```python
from build123d import *

# Parameters (mm, degrees)
SKETCH1_R           = 18
BOSS_EXTRUDE1_DEPTH = 1.5
SKETCH2_R           = 17.5
BOSS_EXTRUDE2_DEPTH = 1.5
SKETCH3_R           = 12
BOSS_EXTRUDE3_DEPTH = 1
SKETCH4_R           = 10.5
BOSS_EXTRUDE4_DEPTH = 12
SKETCH5_R           = 9.5
BOSS_EXTRUDE5_DEPTH = 1
SKETCH6_R           = 10.5
BOSS_EXTRUDE6_DEPTH = 1
SKETCH8_R           = 2.705
CUT_EXTRUDE1_DEPTH  = 32.176914536
SKETCH9_R           = 7
SKETCH9_R_2         = 5
CUT_EXTRUDE3_DEPTH  = 4
SKETCH10_R          = 1.4
CUT_EXTRUDE4_DEPTH  = 5
CIRPATTERN1_COUNT   = 8


with BuildPart() as part:
    # Sketch1 → Boss-Extrude1 (new body)
    with BuildSketch(Plane(origin=(0, 0, 0), x_dir=(1, 0, 0), z_dir=(0, 1, 0))):
        with Locations(Location((0, 0, 0), (0, 0, 270))):
            Circle(SKETCH1_R)
    extrude(amount=BOSS_EXTRUDE1_DEPTH)

    # Sketch2 → Boss-Extrude2 (add)
    with BuildSketch(Plane.XZ):
        with Locations(Location((0, 0, 0), (0, 0, 270))):
            Circle(SKETCH2_R)
    extrude(amount=BOSS_EXTRUDE2_DEPTH)

    # Sketch3 → Boss-Extrude3 (add)
    with BuildSketch(Plane.XZ.offset(1.5)):
        with Locations(Location((0, 0, 0), (0, 0, 270))):
            Circle(SKETCH3_R)
    extrude(amount=BOSS_EXTRUDE3_DEPTH)

    # Sketch4 → Boss-Extrude4 (add)
    with BuildSketch(Plane.XZ.offset(2.5)):
        with Locations(Location((0, 0, 0), (0, 0, 270))):
            Circle(SKETCH4_R)
    extrude(amount=BOSS_EXTRUDE4_DEPTH)

    # Sketch5 → Boss-Extrude5 (add)
    with BuildSketch(Plane.XZ.offset(14.5)):
        with Locations(Location((0, 0, 0), (0, 0, 270))):
            Circle(SKETCH5_R)
    extrude(amount=BOSS_EXTRUDE5_DEPTH)

    # Sketch6 → Boss-Extrude6 (add)
    with BuildSketch(Plane.XZ.offset(15.5)):
        with Locations(Location((0, 0, 0), (0, 0, 270))):
            Circle(SKETCH6_R)
    extrude(amount=BOSS_EXTRUDE6_DEPTH)

    # Sketch7 → Cut-Revolve1 (revolve, cut)
    with BuildSketch(Plane.XY):
        with BuildLine():
            Line((-8.5, -16.5), (0, -16.5))
            Line((0, -16.5), (0, -8))
            ThreePointArc((0, -8), (-6.01040764, -10.48959236), (-8.5, -16.5))
        make_face()
    revolve(axis=Axis((0, -16.5, 0), (0, 1, 0)), mode=Mode.SUBTRACT)

    # Sketch8 → Cut-Extrude1 (cut, through all)
    with BuildSketch(Plane(origin=(0, 1.5, 0), x_dir=(1, 0, 0), z_dir=(0, 1, 0))):
        with Locations(Location((0, 0, 0), (0, 0, 270))):
            Circle(SKETCH8_R)
    extrude(amount=-CUT_EXTRUDE1_DEPTH, mode=Mode.SUBTRACT)

    # Sketch9 → Cut-Extrude3 (cut)
    with BuildSketch(Plane(origin=(0, 1.5, 0), x_dir=(1, 0, 0), z_dir=(0, 1, 0))):
        with Locations(Location((0, 0, 0), (0, 0, 270))):
            Circle(SKETCH9_R)
        with Locations(Location((0, 0, 0), (0, 0, 270))):
            Circle(SKETCH9_R_2, mode=Mode.SUBTRACT)
    extrude(amount=-CUT_EXTRUDE3_DEPTH, mode=Mode.SUBTRACT)

    # Sketch10 → Cut-Extrude4 (cut)
    with BuildSketch(Plane(origin=(0, 1.5, 0), x_dir=(1, 0, 0), z_dir=(0, 1, 0))):
        with Locations(Location((0, 15, 0), (0, 0, 270))):
            Circle(SKETCH10_R)
    cut_extrude4 = extrude(amount=-CUT_EXTRUDE4_DEPTH, mode=Mode.SUBTRACT)

    # CirPattern1: Cut-Extrude4 ×8 about axis
    cirpattern1_axis = Axis((0, 0, 0), (0, 1, 0))
    for i in range(1, CIRPATTERN1_COUNT):
        add(cut_extrude4.rotate(cirpattern1_axis, i * 360 / CIRPATTERN1_COUNT), mode=Mode.SUBTRACT)


solid = part.part
```
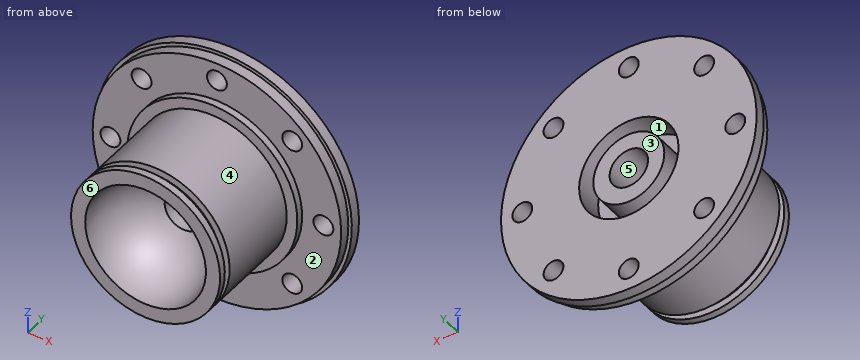
Design review of the part built by this model. Coordinates are the model's own, in mm. Face numbers are marked on the shaded views. A direction names the side the tool comes from. Coordinates: 2 decimals unless noted, no trailing zeros. Order: outer loops, then holes, each group sorted by start corner. A loop starts at its lowest first (then second) coordinate and runs counter-clockwise, first axis right, second up. Notation, with made-up numbers: (80, 43) - (94, 43) arc R28 cw to (94, 72) - close; hole circle Ø9 at (9, 28). An arc over 180 degrees is marked (long way). Answer in a Markdown table with one row per item.
(1) For the marked faces 1, 2 and 3, list the 3-axis set-ups (+Z, -Z, +X, -X, +Y, -Y) from which the entire face can be reached by the end or side of a thin tool; tool diameter is ignored.
Checked values:
| item | result |
|---|---|
| face 1 | +Y |
| face 2 | -Y |
| face 3 | +Z, -Z, +X, -X, +Y |
(2) Wall thickness on line 1 along Y through (x, z) = (-2, 14); line 2 along Z through (x, y) = (2, -0.75); line 3 along X through (y, z) = (-1.25, 16): over which ranges is each line inside the solid? List them lowest first. Write a range as from..to.
Checked values:
| item | result |
|---|---|
| line 1 | -1.5..1.5 |
| line 2 | -17.39..-6.71, -4.58..-1.82, 1.82..4.58, 6.71..17.39 |
| line 3 | -7.09..-0.98, 0.98..7.09 |
(3) Consider section B-B on z = -15. State the section outline as (x, y) points, plus the area to 3 significant figures.
Checked values:
| item | result |
|---|---|
| outline | (-9.95, 0) - (-9.01, 0) - (-9.01, -1.5) - (-1.4, -1.5) - (-1.4, 1.5) - (-9.95, 1.5) - close; (1.4, -1.5) - (9.01, -1.5) - (9.01, 0) - (9.95, 0) - (9.95, 1.5) - (1.4, 1.5) - close |
| area | 48.5 mm^2 |
(4) Clearance check with flat-ended pins moving along their axes: pin 1 (2.5 mm diameter, centred on x = -15, z = 0, fed in from -Y); pin 2 (3 mm diameter, centred on x = 0, z = -15, fed in from -Y); pin 3 (2 mm diameter, centred on y = -14, z = -1.5, fed in from +X); pin 4 (6 mm diameter, centred on x = 0, z = 0, fed in from -Y). State where each tip first meets the part, or that it passes through.
Checked values:
| item | result |
|---|---|
| pin 1 | through |
| pin 2 | y = -1.5 |
| pin 3 | x = 10.49 |
| pin 4 | y = -8.55 |
(5) The part is to be moulded in two halves that separate along X. For the marked faces 4, 5 and 6, say which applies: released by +X, released by -X, zero draft, split by the parting line, or undercut.
Checked values:
| item | result |
|---|---|
| face 4 | split by the parting line |
| face 5 | undercut |
| face 6 | zero draft |
(6) Consider section A-A on x = -15. State the section outline as (y, z) points, plus the area to 3 significant figures.
Checked values:
| item | result |
|---|---|
| outline | (-1.5, -9.01) - (0, -9.01) - (0, -9.95) - (1.5, -9.95) - (1.5, -1.4) - (-1.5, -1.4) - close; (-1.5, 1.4) - (1.5, 1.4) - (1.5, 9.95) - (0, 9.95) - (0, 9.01) - (-1.5, 9.01) - close |
| area | 48.5 mm^2 |
(7) Consider section C-C on x = 0. Give the number of separate pieces and of enclosed holes in the cut face, plus the area to 3 significant figures.
Checked values:
| item | result |
|---|---|
| separate pieces | 4 |
| enclosed holes | 0 |
| area | 224 mm^2 |
